from build123d import *

# Parameters (mm, degrees)
F1_DEPTH = 1270
F2_R     = 101.6
F3_DEPTH = 1270.001


with BuildPart() as f1:
    # F0 (on Top) → F1 (new body)
    with BuildSketch(Plane.XY):
        with BuildLine():
            ThreePointArc((134.883327, 76.2), (-77.459589, 294.592955), (0, 0))
            Line((0, 0), (1016, 0))
            Line((1016, 0), (1016, 76.2))
            Line((1016, 76.2), (134.883327, 76.2))
        make_face()
    extrude(amount=F1_DEPTH)

    # F2 (on face) → F3 (cut, through all)
    with BuildSketch(Plane.XY.offset(1270)):
        with Locations((0, 157.48)):
            Circle(F2_R)
    extrude(amount=-F3_DEPTH, mode=Mode.SUBTRACT)


solid = f1.part
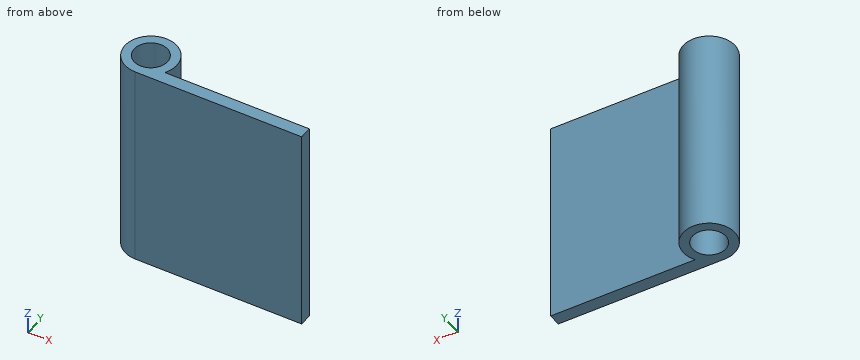
Read the model definition and answer for the solid it produces. Units are mm, in the model's axes. Round coordinates to 2 decimals unless told otherwise and drop trailing zeros. Write each loop counter-clockwise with the first axis right and the second up, starting at its lowest first coordinate (ties: lowest second). Pieces come first, ordered by that corner, then holes.
1. The part is cut by section C-C, the plane x = 365. Determine the outline of the cut face in (y, z), then the cut area to 3 significant figures.
2. The part is cut by section B-B, the plane z = 688. Determine the outline of the cut face in (x, y), then the cut area to 3 significant figures.
3. Straight lines are drawn through the part: L1, parallel to Y at x = 0, z = 731.5; L2, parallel to X at y = 164.5, z = 1120; L3, parallel to X at y = 157, z = 563. For each, find the intervals that lie inside material, in ascending order.
4. Given pin 1 Ø3 at (y, z) = (180, 273) entering from -X; pin 2 Ø2 at (x, y) = (766.5, 66.5) entering from -Z, each flat-ended and moving along its own axis, determine where each tip first touches the part or whether it passes through.
5. The part is cut by section A-A, the plane y = 157.48. Determine the outline of the cut face in (x, z), then the cut area to 3 significant figures.
Values:
1. outline: (0, 0) - (76.2, 0) - (76.2, 1270) - (0, 1270) - close
1. area: 96,800 mm2
2. outline: (0, 0) - (1016, 0) - (1016, 76.2) - (134.88, 76.2) arc R157.48 ccw (long way) to start; hole circle Ø203.2 at (0, 157.48)
2. area: 116,000 mm2
3. L1: y = 0 to 55.88, 259.08 to 314.96
3. L2: x = -157.32 to -101.36, 101.36 to 157.32
3. L3: x = -157.48 to -101.6, 101.6 to 157.48
4. pin 1: stops at x = -156.07
4. pin 2: stops at z = 0
5. outline: (-157.48, 0) - (-101.6, 0) - (-101.6, 1270) - (-157.48, 1270) - close; (101.6, 0) - (157.48, 0) - (157.48, 1270) - (101.6, 1270) - close
5. area: 142,000 mm2
